Autodesk Inventor part; units mm, degrees
ref_plane "YZ Plane" through (0, 0, 0) normal (1, 0, 0) x (0, 1, 0)
ref_plane "XZ Plane" through (0, 0, 0) normal (0, 1, 0) x (-1, 0, 0)
ref_plane "XY Plane" through (0, 0, 0) normal (0, 0, 1) x (1, 0, 0)
sketch "Esquisse2" plane through (0, 0, 0) normal (0, 0, 1) x (1, 0, 0)
  line L0 (10, 110) -> (50, 110)
  line L1 (50, 110) -> (50, 10)
  line L2 (50, 10) -> (10, 10)
  line L3 (10, 10) -> (10, 110)
  line L4 (0, 132) -> (0, -22) construction
  line L5 (-10, 0) -> (60, 0) construction
  point P0 (0, 0)
  dimension "d0" = 40
  dimension "d1" = 100
  dimension "d2" = 10
  dimension "d3" = 10
extrude "Extrusion1" add sketch "Esquisse2" along normal blind 6
sketch "Esquisse3" plane through (0, 0, 6) normal (0, 0, 1) x (1, 0, 0)
  line L0 (50, 10) -> (50, 110) construction
  line L1 (50, 110) -> (10, 110) construction
  line L2 (10, 110) -> (10, 10) construction
  line L3 (10, 10) -> (50, 10) construction
  line L4 (50, 10) -> (10, 10)
  line L5 (10, 10) -> (10, 16)
  line L6 (10, 16) -> (50, 16)
  line L7 (50, 16) -> (50, 10)
  point P0 (0, 0)
  dimension "d6" = 6
extrude "Extrusion2" add sketch "Esquisse3" along normal blind 50
sketch "Esquisse4" plane through (0, 0, 0) normal (0, 0, -1) x (-1, 0, 0)
  line L0 (-50, 10) -> (-50, 110) construction
  line L1 (-10, 10) -> (-50, 10) construction
  line L2 (-10, 110) -> (-10, 10) construction
  line L3 (-50, 110) -> (-10, 110) construction
  line L4 (-10, 110) -> (-50, 110) construction
  line L5 (-50, 110) -> (-50, 65) construction
  line L6 (-50, 65) -> (-10, 65) construction
  line L7 (-10, 65) -> (-10, 110) construction
  circle A0 centre (-30, 87.5) radius 3
  point P0 (0, 0)
  dimension "d9" = 45
  dimension "d10" = 6
  dimension "d11" = 20
  dimension "d12" = 22.5
hole "Perçage1" at (30, 87.5, 0) direction (0, 0, 1) diameter 6 depth 6
sketch "Esquisse5" plane through (10, 10, 0) normal (0, -1, 0) x (1, 0, 0)
  line L0 (0, 0) -> (40, 0) construction
  line L1 (40, 0) -> (40, 56) construction
  line L2 (0, 56) -> (40, 56) construction
  line L3 (0, 0) -> (0, 56) construction
  line L4 (50, 56) -> (-10, 56)
  line L5 (-10, 56) -> (-10, 0)
  line L6 (-10, 0) -> (50, 0)
  line L7 (50, 0) -> (50, 56)
  line L8 (0, 56) -> (40, 56) construction
  point P0 (-10, 0)
  dimension "d20" = 60
  dimension "d21" = 10
extrude "Extrusion3" add sketch "Esquisse5" against normal blind 6
sketch "Esquisse6" plane through (0, 0, 0) normal (0, 0, -1) x (-1, 0, 0)
  line L0 (-10, 110) -> (-10, 16) construction
  line L1 (-50, 110) -> (-10, 110) construction
  line L2 (-50, 16) -> (-50, 110) construction
  line L3 (-60, 16) -> (-50, 16) construction
  line L4 (-60, 10) -> (-60, 16) construction
  line L5 (0, 10) -> (-60, 10) construction
  line L6 (0, 10) -> (0, 16) construction
  line L7 (-10, 16) -> (0, 16) construction
  circle A0 centre (-30, 87.5) radius 3 construction
  line L8 (0, 16) -> (-10, 30)
  line L9 (-60, 16) -> (-50, 30)
  line L10 (0, 16) -> (-10, 16)
  line L11 (-10, 16) -> (-10, 30)
  line L12 (-50, 30) -> (-50, 16)
  line L13 (-60, 16) -> (-50, 16)
  point P0 (0, 0)
  dimension "d24" = 14
  dimension "d25" = 14
extrude "Extrusion4" add sketch "Esquisse6" against normal blind 6
sketch "Sketch7" plane through (50, 110, 6) normal (1, 0, 0) x (0, 0, -1)
  point P0 (6, -110)
fillet "Fillet1" radius 20 1 edges at (30, 16, 6)
properties part number "P005_supportCapteursTripod"
Can you work these out from the model? Positions are in its coordinate system, mm. A direction names the side the tool comes from. Coordinates: 2 decimals unless noted, no trailing zeros. Write each loop counter-clockwise with the first axis right and the second up, starting at its lowest first coordinate (ties: lowest second). Pieces come first, ordered by that corner, then holes. Notation, with made-up numbers: (-15.5, 18) -> (24.5, 18) arc R21 cw to (24.5, 41) -> close; hole circle Ø3 at (81.5, 0.5). An arc over 180 degrees is marked (long way). Answer as CSV lines item,"result".
1) On a 3-axis mill with a long thin cutter (end or side, diameter ignored), from which of +Z, -Z, +X, -X, +Y, -Y can I reach the whole of each face in a straight line? I mean faces 1 (the cylindrical face through (29.9, 84.5, 3)), 2 (the flat face through (0, 13, 28)), 3 (the flat face through (50, 71, 3)), 4 (the flat face through (10, 69, 3)), 5 (the flat face through (30, 16, 41)). Say none if no direction works.
Check result:
face 1,"+Z, -Z"
face 2,"+Z, -Z, -X, +Y, -Y"
face 3,"+Z, -Z, +X, +Y"
face 4,"+Z, -Z, -X, +Y"
face 5,"+Z, +X, -X, +Y"
2) If I drill on line 1 (Y direction, x = 30, z = 1.9); line 2 (Y direction, x = 37, z = 47.5); line 3 (X direction, y = 87, z = 3), over which ranges is the centre line in solid material (lowest first)? Write a range as from..to.
Check result:
line 1,"10..84.5, 90.5..110"
line 2,"10..16"
line 3,"10..27.04, 32.96..50"
3) Will these pins go through, and if not, where does the flat tip stop? P1, Ø1, axis at x = 6.5, z = 12, coming from the +Y side (3 decimals); P2, Ø5.5, axis at y = 71.5, z = 3, coming from the -X side; P3, Ø7.5, axis at y = 56, z = 3.5, coming from the +X side.
Check result:
P1,"y = 22.225"
P2,"x = 10"
P3,"x = 50"
4) If we section it at B-B on x = 30: Please give me the cut outline in (y, z), then the cut area to 3 significant figures.
Check result:
outline,"(10, 0) -> (84.5, 0) -> (84.5, 6) -> (36, 6) arc R20 cw to (16, 26) -> (16, 56) -> (10, 56) -> close; (90.5, 0) -> (110, 0) -> (110, 6) -> (90.5, 6) -> close"
area,"950 mm²"
5) If we section it at A-A on y = 87.5: Please give me the cut outline in (x, z).
Check result:
outline,"(10, 0) -> (27, 0) -> (27, 6) -> (10, 6) -> close; (33, 0) -> (50, 0) -> (50, 6) -> (33, 6) -> close"
6) If we section it at D-D on x = 56: Please give me the cut outline in (y, z), then the cut area to 3 significant figures.
Check result:
outline,"(10, 0) -> (21.6, 0) -> (21.6, 12.12) arc R20 cw to (16, 26) -> (16, 56) -> (10, 56) -> close"
area,"428 mm²"
7) If we section it at C-C on z = 45: Please give me the cut outline in (x, y).
Check result:
outline,"(0, 10) -> (60, 10) -> (60, 16) -> (0, 16) -> close"
